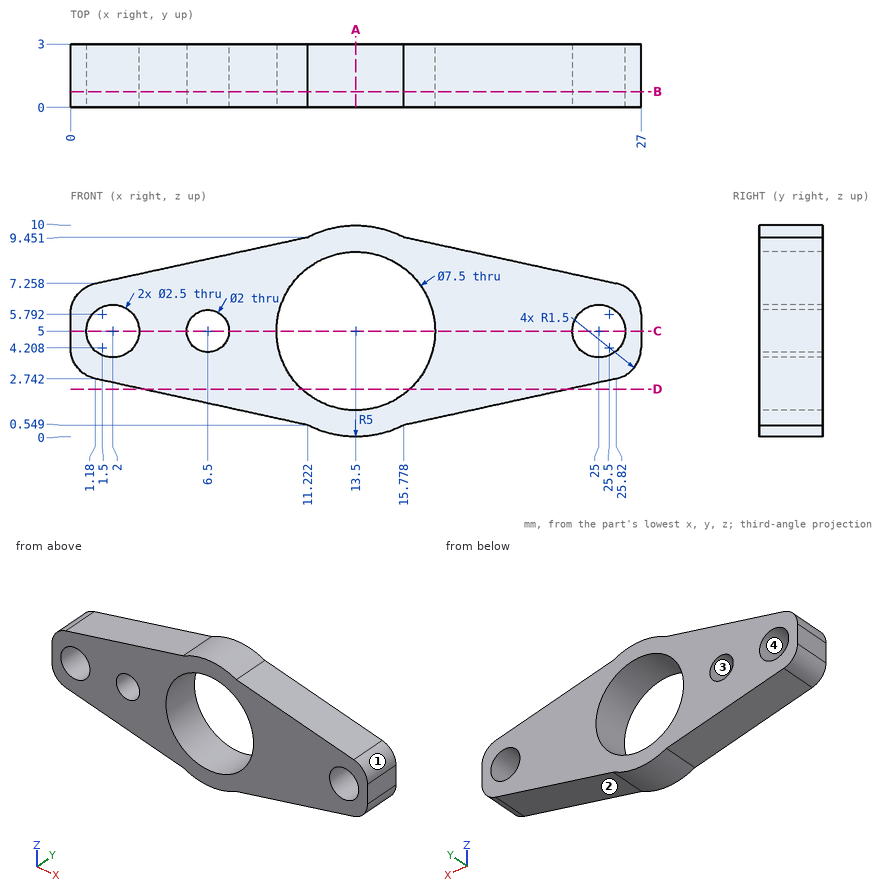
Verification items for this drawing (mm, ordinates from the low corner). Round coordinates to 2 decimals unless told otherwise and drop trailing zeros. Write each loop counter-clockwise with the first axis right and the second up, starting at its lowest first coordinate (ties: lowest second). Pieces come first, ordered by that corner, then holes. Notation, with made-up numbers: M 36.5,18.25 L 92.5,18.25 A27 ccw 92.5,48.25 Z; hole C -19,-18.75 d3. An arc over 180 degrees is marked long. Write item = value, one per line. Start each with the question number.
1. Section check D-D, the plane z = 2.25. Record the cut outline in (x, y).
2. Section check C-C, the plane z = 5. Record the cut outline in (x, y).
3. Gauge pin test, flat end, axial feed: pin 1 (1.6 mm diameter, centred on x = 6.5, z = 5, fed in from -Y). Record the tip position at first contact, or that the pin passes through.
4. Scan lines: line 1 (X direction, y = 1.8, z = 5); line 2 (Z direction, x = 13.5, y = 0.85); line 3 (Z direction, x = 2, y = 1.35). Record each from-to range of solid material in increasing order. Write a range as [from, to].
5. Release check for a two-part mould opening along Z. For the marked faces 1, 2, 3 and 4 record: pulls with the +Z half, pulls with the -Z half, needs draft (parallel to the pull), parting line crosses it, or undercut.
6. Section check A-A, the plane x = 13.5. Record the cut outline in (y, z).
7. Section check B-B, the plane y = 0.75. Record the cut outline in (x, z).
Results found:
q1.outline = M 3.43,0 L 10.95,0 L 10.95,3 L 3.43,3 Z; M 16.05,0 L 23.57,0 L 23.57,3 L 16.05,3 Z
q2.outline = M 0,0 L 0.75,0 L 0.75,3 L 0,3 Z; M 3.25,0 L 5.5,0 L 5.5,3 L 3.25,3 Z; M 7.5,0 L 9.75,0 L 9.75,3 L 7.5,3 Z; M 17.25,0 L 23.75,0 L 23.75,3 L 17.25,3 Z; M 26.25,0 L 27,0 L 27,3 L 26.25,3 Z
q3.pin_1 = through
q4.line_1 = [0, 0.75], [3.25, 5.5], [7.5, 9.75], [17.25, 23.75], [26.25, 27]
q4.line_2 = [0, 1.25], [8.75, 10]
q4.line_3 = [2.56, 3.75], [6.25, 7.44]
q5.face_1 = pulls with the +Z half
q5.face_2 = pulls with the -Z half
q5.face_3 = undercut
q5.face_4 = undercut
q6.outline = M 0,0 L 3,0 L 3,1.25 L 0,1.25 Z; M 0,8.75 L 3,8.75 L 3,10 L 0,10 Z
q7.outline = M 0,4.21 A1.5 ccw 1.18,2.74 L 11.22,0.55 A5 ccw 15.78,0.55 L 25.82,2.74 A1.5 ccw 27,4.21 L 27,5.79 A1.5 ccw 25.82,7.26 L 15.78,9.45 A5 ccw 11.22,9.45 L 1.18,7.26 A1.5 ccw 0,5.79 Z; hole C 2,5 d2.5; hole C 6.5,5 d2; hole C 13.5,5 d7.5; hole C 25,5 d2.5
